Autodesk Fusion 360 part; units mm, degrees
sketch "Sketch1" plane through (0, 0, 0) normal (0, 1, 0) x (1, 0, 0)
  circle A0 centre (0, 0) radius 25.875
  circle A1 centre (0, 0) radius 40
  dimension "d1" = 51.75
  dimension "d2" = 80
extrude "Extrude1" add sketch "Sketch1" along normal blind 15 contours A0
extrude "Extrude2" add sketch "Sketch1" against normal blind 6 contours A0 | A1
sketch "Sketch2" plane through (0, 15, 0) normal (0, 1, 0) x (-1, 0, 0)
  circle A0 centre (0, 0) radius 25.875
  circle A1 centre (0, 0) radius 15.125
  dimension "d7" = 30.25
extrude "Extrude3" cut sketch "Sketch2" against normal blind 77.834 contours A1
sketch "Sketch3" plane through (0, 15, 0) normal (0, 1, 0) x (-1, 0, 0)
  circle A0 centre (0, 0) radius 15.125
  circle A1 centre (0, 0) radius 25.875
  circle A2 centre (0, 0) radius 21.5
  dimension "d10" = 43
extrude "Extrude4" cut sketch "Sketch3" against normal blind 9 contours A2
chamfer "Chamfer1" distance 2 angle 45 1 edges at (14.1015, -6, -5.4694)
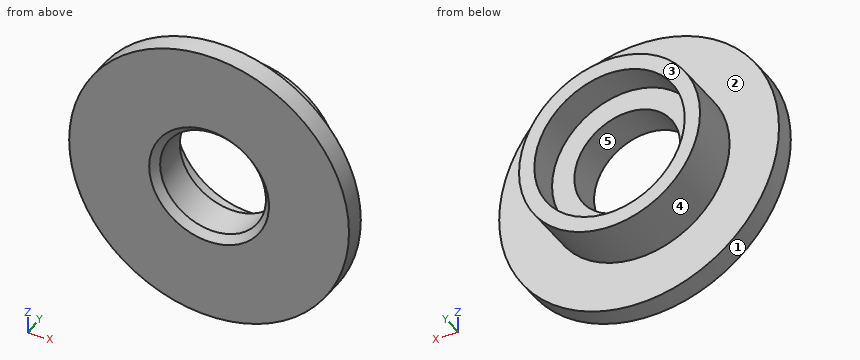
Model file for the job. Use its own axes, mm. Face numbers are marked on the shaded views. A direction names the side the tool comes from. Give positions to 0.01 mm unless a question says otherwise; leave off trailing zeros. Order: outer loops, then holes, each group sorted by start corner. A loop starts at its lowest first (then second) coordinate and runs counter-clockwise, first axis right, second up. Notation, with made-up numbers: M 56.25,33.5 L 75.25,33.5 A14 cw 75.25,52.5 Z; hole C -17.75,-4 d6. An arc over 180 degrees is marked long. Write item = value, one per line.
Q1. Cut at D-D, the plane y = -2.25. List the corners of the cut face in (x, z) (3 decimals).
Derived:
outline = C 0,0 d80; hole C 0,0 d30.25
Q2. Two-plate mould, pull along X, no slides. Class the marked faces 3, 4 and 5: pulls with the +X half, pulls with the -X half, needs draft (parallel to the pull), parting line crosses it, or undercut.
Derived:
face_3 = needs draft
face_4 = parting line crosses it
face_5 = undercut
Q3. Drill centre lines: line 1 (Z direction, x = 0.5, y = 4.25); line 2 (Z direction, x = 0, y = 10.5) (3 decimals); line 3 (X direction, y = 14.25, z = 17). Where is each one in solid material? Low to high. Write a range as [from, to].
Derived:
line_1 = [-25.87, -15.12], [15.12, 25.87]
line_2 = [-25.875, -21.5], [21.5, 25.875]
line_3 = [-19.51, -13.16], [13.16, 19.51]
Q4. Flat gauge pins, fed straight in: pin 1 (1.5 mm diameter, centred on y = 3, z = 7.5, fed in from +X); pin 2 (6 mm diameter, centred on x = -14, y = 1.5, fed in from -Z); pin 3 (3 mm diameter, centred on y = 3, z = -14, fed in from +X); pin 4 (1.5 mm diameter, centred on y = 5, z = -28, fed in from +X). Where does each tip first touch, or does it go through?
Derived:
pin_1 = 24.98
pin_2 = -38.34
pin_3 = 22.66
pin_4 = through
Q5. Cut at B-B, the plane x = 0. List the corners of the cut face in (y, z) (3 decimals), then the cut area to 3 significant figures.
Derived:
outline = M -6,-40 L 0,-40 L 0,-25.875 L 15,-25.875 L 15,-21.5 L 6,-21.5 L 6,-15.125 L -4,-15.125 L -6,-17.125 Z; M -6,17.125 L -4,15.125 L 6,15.125 L 6,21.5 L 15,21.5 L 15,25.875 L 0,25.875 L 0,40 L -6,40 Z
area = 502 mm2
Q6. Cut at A-A, the plane z = 0. List the corners of the cut face in (x, y) (3 decimals).
Derived:
outline = M -40,-6 L -17.125,-6 L -15.125,-4 L -15.125,6 L -21.5,6 L -21.5,15 L -25.875,15 L -25.875,0 L -40,0 Z; M 15.125,-4 L 17.125,-6 L 40,-6 L 40,0 L 25.875,0 L 25.875,15 L 21.5,15 L 21.5,6 L 15.125,6 Z
Q7. Tool access for the marked faces 1 and 2: list every direction of +Z, -Z, +X, -X, +Y, -Y with a clear straight run to the whole face (end or side of a thin tool).
Derived:
face_1 = +Y, -Y
face_2 = +Y
Q8. Cut at C-C, the plane y = 2. List the corners of the cut face in (x, z) (3 decimals).
Derived:
outline = C 0,0 d51.75; hole C 0,0 d30.25
